The model under review builds one solid part; all positions refer to its coordinate system, in mm. Round coordinates to 2 decimals unless told otherwise and drop trailing zeros. Order: outer loops, then holes, each group sorted by start corner. A loop starts at its lowest first (then second) coordinate and runs counter-clockwise, first axis right, second up.
from build123d import *

# Parameters (mm, degrees)
SKETCH2_W           = 95.25
SKETCH2_H           = 419.1
BOSS_EXTRUDE1_DEPTH = 6.35
SKETCH3_W           = 6.35
SKETCH3_H           = 12.7
CUT_EXTRUDE1_DEPTH  = 7.35
LPATTERN1_COUNT     = 17
LPATTERN1_PITCH     = 25.4
SKETCH4_W           = 12.7
SKETCH4_H           = 6.35
CUT_EXTRUDE2_DEPTH  = 7.35
SKETCH5_W           = 6.35
SKETCH5_H           = 12.7
CUT_EXTRUDE3_DEPTH  = 7.35
LPATTERN2_COUNT     = 4
LPATTERN2_PITCH     = 25.4
SKETCH6_W           = 12.7
SKETCH6_H           = 6.35
CUT_EXTRUDE4_DEPTH  = 7.35
LPATTERN3_COUNT     = 2
LPATTERN3_PITCH     = 25.4
LPATTERN3_COL_COUNT = 2
LPATTERN3_COL_PITCH = 25.4


with BuildPart() as part:
    # Sketch2 → Boss-Extrude1 (new body)
    with BuildSketch(Plane.XY):
        with Locations((47.625, 209.55)):
            Rectangle(SKETCH2_W, SKETCH2_H)
    extrude(amount=BOSS_EXTRUDE1_DEPTH)

    # Sketch3 → Cut-Extrude1 (cut, through all)
    with BuildSketch(Plane.XY.offset(6.35)):
        with Locations((3.175, 6.35)):
            Rectangle(SKETCH3_W, SKETCH3_H)
        with Locations((92.075, 6.35)):
            Rectangle(SKETCH3_W, SKETCH3_H)
    cut_extrude1 = extrude(amount=-CUT_EXTRUDE1_DEPTH, mode=Mode.SUBTRACT)

    # LPattern1: Cut-Extrude1 ×17
    with Locations(*[(0, i * LPATTERN1_PITCH, 0) for i in range(1, LPATTERN1_COUNT)]):
        add(cut_extrude1, mode=Mode.SUBTRACT)

    # Sketch4 → Cut-Extrude2 (cut, through all)
    with BuildSketch(Plane.XY.offset(6.35)):
        with Locations((47.625, 415.925)):
            Rectangle(SKETCH4_W, SKETCH4_H)
        with Locations((22.225, 415.925)):
            Rectangle(SKETCH4_W, SKETCH4_H)
        with Locations((73.025, 415.925)):
            Rectangle(SKETCH4_W, SKETCH4_H)
    extrude(amount=-CUT_EXTRUDE2_DEPTH, mode=Mode.SUBTRACT)

    # Sketch5 → Cut-Extrude3 (cut, through all)
    with BuildSketch(Plane.XY.offset(6.35)):
        with Locations((9.525, 6.35)):
            Rectangle(SKETCH5_W, SKETCH5_H)
        with Locations((85.725, 6.35)):
            Rectangle(SKETCH5_W, SKETCH5_H)
    cut_extrude3 = extrude(amount=-CUT_EXTRUDE3_DEPTH, mode=Mode.SUBTRACT)

    # LPattern2: Cut-Extrude3 ×4
    with Locations(*[(0, i * LPATTERN2_PITCH, 0) for i in range(1, LPATTERN2_COUNT)]):
        add(cut_extrude3, mode=Mode.SUBTRACT)

    # Sketch6 → Cut-Extrude4 (cut, through all)
    with BuildSketch(Plane.XY.offset(6.35)):
        with Locations((47.625, 142.875)):
            Rectangle(SKETCH6_W, SKETCH6_H)
    cut_extrude4 = extrude(amount=-CUT_EXTRUDE4_DEPTH, mode=Mode.SUBTRACT)

    # LPattern3: Cut-Extrude4 ×2
    with Locations(*[(i * LPATTERN3_PITCH, 0, 0) for i in range(1, LPATTERN3_COUNT)]):
        add(cut_extrude4, mode=Mode.SUBTRACT)

    # LPattern3 col: Cut-Extrude4 ×2
    with Locations(*[(-i * LPATTERN3_COL_PITCH, 0, 0) for i in range(1, LPATTERN3_COL_COUNT)]):
        add(cut_extrude4, mode=Mode.SUBTRACT)


solid = part.part
(1) Clearance check with flat-ended pins moving along their axes: P1, Ø3, axis at y = 235.5, z = 2, coming from the +X side; P2, Ø1.9, axis at x = 3, z = 1.5, coming from the -Y side. State where each tip first meets the part, or that it passes through.
(2) We need section A-A (x = 22). Give the boundary of the cut face in (y, z), and give its area (3 significant figures).
(3) We need section B-B (z = 1.25). Count the separate pieces of the cut face and the enclosed holes in it, and give its area (3 significant figures).
(4) We need section C-C (y = 108.5). Give the boundary of the cut face in (x, z), and give its area (3 significant figures).
(5) To check wall thickness, follow L1, parallel to X at y = 143.5, z = 6.25 (3 decimals); L2, parallel to Y at x = 87, z = 6.25; L3, parallel to Y at x = 75.5, z = 3.5. State the ranges of each line that lie inside material, in increasing order.
Verdict:
1. P1: stops at x = 88.9
1. P2: stops at y = 12.7
2. outline: (0, 0) - (139.7, 0) - (139.7, 6.35) - (0, 6.35) - close; (146.05, 0) - (412.75, 0) - (412.75, 6.35) - (146.05, 6.35) - close
2. area: 2,580 mm2
3. separate pieces: 1
3. enclosed holes: 3
3. area: 36,000 mm2
4. outline: (6.35, 0) - (88.9, 0) - (88.9, 6.35) - (6.35, 6.35) - close
4. area: 524 mm2
5. L1: x = 0 to 15.875, 28.575 to 41.275, 53.975 to 66.675, 79.375 to 95.25
5. L2: y = 12.7 to 25.4, 38.1 to 50.8, 63.5 to 76.2, 88.9 to 419.1
5. L3: y = 0 to 139.7, 146.05 to 412.75
